Read the model definition and answer for the solid it produces. Units are mm, in the model's axes. Coordinates: 2 decimals unless noted, no trailing zeros. Write each loop counter-clockwise with the first axis right and the second up, starting at its lowest first coordinate (ties: lowest second). Pieces come first, ordered by that corner, then holes. Notation, with made-up numbers: (82, 60) - (99, 60) arc R25 cw to (99, 86) - close; hole circle Ø9 at (-6.5, 43). An arc over 180 degrees is marked (long way). Use a Markdown table: item, result.
from build123d import *

# Parameters (mm, degrees)
SKETCH1_W            = 274.7772
SKETCH1_H            = 114.4016
BOSS_EXTRUDE1_DEPTH  = 6.35
M3_CLEARANCE_HOLE1_D = 3.4
CUT_EXTRUDE2_DEPTH   = 298.708848075


with BuildPart() as part:
    # Sketch1 → Boss-Extrude1 (new body)
    with BuildSketch(Plane.XY):
        with Locations((137.3886, 57.2008)):
            Rectangle(SKETCH1_W, SKETCH1_H)
    extrude(amount=BOSS_EXTRUDE1_DEPTH)

    # M3 Clearance Hole1 (through all)
    with Locations(Plane.XY.offset(6.35)):
        with Locations((12.3444, 92.4052), (12.3444, 19.3802), (262.4328, 54.3052), (262.4328, 92.4052)):
            Hole(M3_CLEARANCE_HOLE1_D / 2)

    # Sketch5 → Cut-Extrude2 (cut, through all)
    with BuildSketch(Plane.XY.offset(6.35)):
        Polygon((0, 0), (274.7772, 0), (274.7772, 38.617417045), align=None)
    extrude(amount=-CUT_EXTRUDE2_DEPTH, mode=Mode.SUBTRACT)


solid = part.part
(1) A cutting plane is placed at B-B, the plane x = 226.5. Write down the section's boundary in (y, z).
Report:
| item | result |
|---|---|
| outline | (31.83, 0) - (114.4, 0) - (114.4, 6.35) - (31.83, 6.35) - close |
(2) A cutting plane is placed at C-C, the plane y = 10. Write down the section's boundary in (x, z), and give its area (3 significant figures).
Report:
| item | result |
|---|---|
| outline | (0, 0) - (71.15, 0) - (71.15, 6.35) - (0, 6.35) - close |
| area | 452 mm² |
(3) Straight lines are drawn through the part: L1, parallel to X at y = 53.5, z = 3.25; L2, parallel to Y at x = 85, z = 2.5; L3, parallel to Y at x = 156.5, z = 0.5. For each, find the intervals that lie inside material, in ascending order.
Report:
| item | result |
|---|---|
| L1 | x = 0 to 260.94, 263.93 to 274.78 |
| L2 | y = 11.95 to 114.4 |
| L3 | y = 21.99 to 114.4 |
(4) A cutting plane is placed at A-A, the plane z = 3. Write down the section's boundary in (x, y).
Report:
| item | result |
|---|---|
| outline | (0, 0) - (274.78, 38.62) - (274.78, 114.4) - (0, 114.4) - close; hole circle Ø3.4 at (12.34, 19.38); hole circle Ø3.4 at (12.34, 92.41); hole circle Ø3.4 at (262.43, 54.31); hole circle Ø3.4 at (262.43, 92.41) |
